Geometry check sheet. Reference: the model listing, model coordinates, mm. Face numbers are marked on the shaded views. A direction names the side the tool comes from. Coordinates: 2 decimals unless noted, no trailing zeros. Loops run counter-clockwise (first coordinate to the right, second up) from the corner with the lowest first, then second, coordinate; pieces in that order, holes last. Notation, with made-up numbers: (86, 3) - (111, 3) arc R10 cw to (111, 17) - close; hole circle Ø9 at (40, 50.5). An arc over 180 degrees is marked (long way). One line per item, written item: value.
Autodesk Inventor part; units mm, degrees
ref_plane "YZ Plane" through (0, 0, 0) normal (1, 0, 0) x (0, 1, 0)
ref_plane "XZ Plane" through (0, 0, 0) normal (0, 1, 0) x (-1, 0, 0)
ref_plane "XY Plane" through (0, 0, 0) normal (0, 0, 1) x (1, 0, 0)
sketch "Sketch1" plane through (0, 0, 0) normal (0, 0, 1) x (1, 0, 0)
  line L0 (0, 60) -> (0, -60)
  line L1 (0, -60) -> (-10, -60)
  line L2 (-10, -60) -> (-10, 60)
  line L3 (-10, 60) -> (0, 60)
  point P0 (0, 0)
  dimension "d27" = 120
  dimension "d28" = 10
extrude "Extrusion1" add sketch "Sketch1" along normal blind 20
sketch "Sketch2" plane through (0, 0, 20) normal (0, 0, 1) x (1, 0, 0)
  line L0 (0, 5) -> (0, -5)
  line L1 (0, -50) -> (0, 50)
  line L2 (0, 5) -> (-55, 5)
  line L3 (-55, 5) -> (-55, -5)
  line L4 (-55, -5) -> (0, -5)
  point P0 (0, 0)
  dimension "d5" = 10
  dimension "d6" = 55
  dimension "d7" = 10
extrude "Extrusion2" add sketch "Sketch2" along normal blind 30
sketch "Sketch3" plane through (-55, 5, 20) normal (0, 1, 0) x (1, 0, 0)
  line L0 (0, 0) -> (0, -30)
  line L1 (0, 0) -> (45, 0)
  line L2 (0, -30) -> (55, -30)
  circle A0 centre (12.5, -15) radius 7.5
  point P0 (55, 20)
  dimension "d12" = 15
extrude "Extrusion3" cut sketch "Sketch3" against normal blind 10
sketch "Sketch6" plane through (0, 0, 20) normal (0, 0, 1) x (1, 0, 0)
  circle A0 centre (-5, -52.5) radius 2.5
  circle A1 centre (-5, 52.5) radius 2.5
  point P0 (0, 0)
  dimension "d29" = 5
  dimension "d30" = 5
extrude "Extrusion6" cut sketch "Sketch6" against normal up to surface (20 mm away)
thread "Thread2"
properties part number "steering_connector[1]" material "Wood (Birch)"
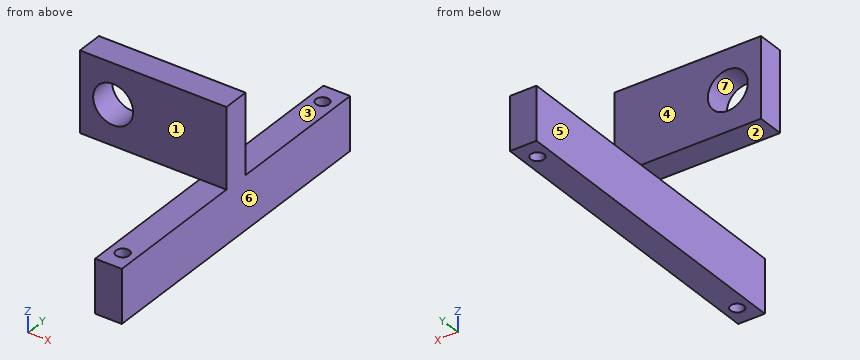
(1) Cross-section at C-C on z = 17.5. Record the cut outline in (x, y).
Reply:
outline: (-10, -60) - (0, -60) - (0, 60) - (-10, 60) - close; hole circle Ø5 at (-5, -52.5); hole circle Ø5 at (-5, 52.5)
(2) Material ranges on probe 1 along Y at (x, z) = (-5, 6.75); probe 2 along Z at (x, y) = (-42.5, 0.75); probe 3 along Y at (x, z) = (-7, 2.5), recorded low to high. Write a range as from..to.
Reply:
probe 1: -60..-55, -50..50, 55..60
probe 2: 20..27.5, 42.5..50
probe 3: -60..-54, -51..51, 54..60
(3) Cross-section at D-D on x = -5. Record the cut outline in (y, z), and give its area (3 significant figures).
Reply:
outline: (-60, 0) - (-55, 0) - (-55, 20) - (-60, 20) - close; (-50, 0) - (50, 0) - (50, 20) - (5, 20) - (5, 50) - (-5, 50) - (-5, 20) - (-50, 20) - close; (55, 0) - (60, 0) - (60, 20) - (55, 20) - close
area: 2,500 mm2
(4) Go/stop test with flat-tipped pins: pin 1 Ø4.5 at (x, y) = (-5, 52.5) entering from -Z; pin 2 Ø12 at (x, y) = (-8.5, -43) entering from +Z; pin 3 Ø17 at (x, z) = (-42.5, 35) entering from +Y; pin 4 Ø9 at (x, z) = (-30.5, 42) entering from -Y. Record where each tip stops, or that it passes through.
Reply:
pin 1: through
pin 2: z = 20
pin 3: y = 5
pin 4: y = -5
(5) Access from +Z, -Z, +X, -X, +Y, -Y to the whole of each face (thin tool, end or side, straight path). Record for the marked faces 1, 2 and 3.
Reply:
face 1: +Z, +X, -X, -Y
face 2: -Z, -X, +Y, -Y
face 3: +Z, +X, -X, +Y
(6) Cross-section at B-B on x = -42.5. Record the cut outline in (y, z), and give its area (3 significant figures).
Reply:
outline: (-5, 20) - (5, 20) - (5, 27.5) - (-5, 27.5) - close; (-5, 42.5) - (5, 42.5) - (5, 50) - (-5, 50) - close
area: 150 mm2
(7) Release check for a two-part mould opening along X. For the marked faces 4, 5, 6 and 7 record: pulls with the +X half, pulls with the -X half, needs draft (parallel to the pull), parting line crosses it, or undercut.
Reply:
face 4: needs draft
face 5: pulls with the -X half
face 6: pulls with the +X half
face 7: undercut
(8) Cross-section at A-A on z = 35. Record the cut outline in (x, y), and give its area (3 significant figures).
Reply:
outline: (-55, -5) - (-50, -5) - (-50, 5) - (-55, 5) - close; (-35, -5) - (0, -5) - (0, 5) - (-35, 5) - close
area: 400 mm2
